```python
from build123d import *

# Parameters (mm, degrees)
SKETCH_1_R          = 5
SKETCH_1_W          = 19.999962028
SKETCH_1_H          = 6.000037038
EXTRUDE_1_DEPTH     = 13
SKETCH_2_R          = 2
CUT_EXTRUDE_1_DEPTH = 36.693120105
SKETCH_3_W          = 1
SKETCH_3_H          = 13
CUT_EXTRUDE_2_DEPTH = 13
FILLET_1_R          = 10


with BuildPart() as part:
    # 草图1 → 凸台-拉伸1 (new body)
    # profile 1 of 10: a face of its own
    with BuildSketch(Plane.XY):
        with BuildLine():
            ThreePointArc((18.008966142, -1.894393619), (10.046238322, 2.288323413), (16.668970702, 8.374337866))
            Line((16.668970702, 8.374337866), (0, 12))
            Line((0, 12), (-16.6689706, 8.374337888))
            ThreePointArc((-16.6689706, 8.374337888), (-12.048865281, 7.282483993), (-10, 3))
            ThreePointArc((-10, 3), (-12.632014098, -1.693043455), (-18.008966133, -1.894393624))
            Line((-18.008966133, -1.894393624), (-9.999981014, -5.999962962))
            Line((-9.999981014, -5.999962962), (9.999981014, -5.999962962))
            Line((9.999981014, -5.999962962), (18.008966142, -1.894393619))
        make_face()
        with Locations(Location((0, 2, 0), (0, 0, 180))):
            Circle(SKETCH_1_R, mode=Mode.SUBTRACT)
    # profile 2 of 10: a face of its own
    with BuildSketch(Plane.XY):
        with BuildLine():
            ThreePointArc((-10, 3), (-12.048865281, 7.282483993), (-16.6689706, 8.374337888))
            ThreePointArc((-16.6689706, 8.374337888), (-18.13580723, 7.827268404), (-19.389087297, 6.889087297))
            Line((-19.389087297, 6.889087297), (-18.680885962, 6.180885962))
            ThreePointArc((-18.680885962, 6.180885962), (-13.778516922, 7.156027793), (-11.001547932, 3))
            ThreePointArc((-11.001547932, 3), (-13.778516922, -1.156027793), (-18.680885962, -0.180885962))
            Line((-18.680885962, -0.180885962), (-19.389087297, -0.889087297))
            ThreePointArc((-19.389087297, -0.889087297), (-18.738276104, -1.445623452), (-18.008966133, -1.894393624))
            ThreePointArc((-18.008966133, -1.894393624), (-12.632014098, -1.693043455), (-10, 3))
        make_face()
    # profile 3 of 10: a face of its own
    with BuildSketch(Plane.XY):
        with BuildLine():
            Line((-18.680885962, 6.180885962), (-19.389087297, 6.889087297))
            ThreePointArc((-19.389087297, 6.889087297), (-20.581337429, 5.104758878), (-21, 3))
            ThreePointArc((-21, 3), (-20.581337429, 0.895241122), (-19.389087297, -0.889087297))
            Line((-19.389087297, -0.889087297), (-18.680885962, -0.180885962))
            ThreePointArc((-18.680885962, -0.180885962), (-19.998452068, 3), (-18.680885962, 6.180885962))
        make_face()
    # profile 4 of 10: a face of its own
    with BuildSketch(Plane.XY):
        with BuildLine():
            ThreePointArc((-10, 3), (-12.048865281, 7.282483993), (-16.6689706, 8.374337888))
            ThreePointArc((-16.6689706, 8.374337888), (-18.13580723, 7.827268404), (-19.389087297, 6.889087297))
            Line((-19.389087297, 6.889087297), (-18.680885962, 6.180885962))
            ThreePointArc((-18.680885962, 6.180885962), (-13.778516922, 7.156027793), (-11.001547932, 3))
            ThreePointArc((-11.001547932, 3), (-13.778516922, -1.156027793), (-18.680885962, -0.180885962))
            Line((-18.680885962, -0.180885962), (-19.389087297, -0.889087297))
            ThreePointArc((-19.389087297, -0.889087297), (-18.738276104, -1.445623452), (-18.008966133, -1.894393624))
            ThreePointArc((-18.008966133, -1.894393624), (-12.632014098, -1.693043455), (-10, 3))
        make_face()
    # profile 5 of 10: a face of its own
    with BuildSketch(Plane.XY):
        with BuildLine():
            Line((-18.680885962, 6.180885962), (-19.389087297, 6.889087297))
            ThreePointArc((-19.389087297, 6.889087297), (-20.581337429, 5.104758878), (-21, 3))
            ThreePointArc((-21, 3), (-20.581337429, 0.895241122), (-19.389087297, -0.889087297))
            Line((-19.389087297, -0.889087297), (-18.680885962, -0.180885962))
            ThreePointArc((-18.680885962, -0.180885962), (-19.998452068, 3), (-18.680885962, 6.180885962))
        make_face()
    # profile 6 of 10: a face of its own
    with BuildSketch(Plane.XY):
        with BuildLine():
            ThreePointArc((18.680885962, -0.180885962), (11.001547932, 3), (18.680885962, 6.180885962))
            Line((18.680885962, 6.180885962), (19.389087297, 6.889087297))
            ThreePointArc((19.389087297, 6.889087297), (18.135807275, 7.82726838), (16.668970702, 8.374337866))
            ThreePointArc((16.668970702, 8.374337866), (10.046238322, 2.288323413), (18.008966142, -1.894393619))
            ThreePointArc((18.008966142, -1.894393619), (18.738276108, -1.445623449), (19.389087297, -0.889087297))
            Line((19.389087297, -0.889087297), (18.680885962, -0.180885962))
        make_face()
    # profile 7 of 10: a face of its own
    with BuildSketch(Plane.XY):
        with BuildLine():
            Line((19.389087297, 6.889087297), (18.680885962, 6.180885962))
            ThreePointArc((18.680885962, 6.180885962), (19.656027793, 4.721483078), (19.998452068, 3))
            ThreePointArc((19.998452068, 3), (19.656027793, 1.278516922), (18.680885962, -0.180885962))
            Line((18.680885962, -0.180885962), (19.389087297, -0.889087297))
            ThreePointArc((19.389087297, -0.889087297), (20.581337429, 0.895241122), (21, 3))
            ThreePointArc((21, 3), (20.581337429, 5.104758878), (19.389087297, 6.889087297))
        make_face()
    # profile 8 of 10: a face of its own
    with BuildSketch(Plane.XY):
        with BuildLine():
            ThreePointArc((18.680885962, -0.180885962), (11.001547932, 3), (18.680885962, 6.180885962))
            Line((18.680885962, 6.180885962), (19.389087297, 6.889087297))
            ThreePointArc((19.389087297, 6.889087297), (18.135807275, 7.82726838), (16.668970702, 8.374337866))
            ThreePointArc((16.668970702, 8.374337866), (10.046238322, 2.288323413), (18.008966142, -1.894393619))
            ThreePointArc((18.008966142, -1.894393619), (18.738276108, -1.445623449), (19.389087297, -0.889087297))
            Line((19.389087297, -0.889087297), (18.680885962, -0.180885962))
        make_face()
    # profile 9 of 10: a face of its own
    with BuildSketch(Plane.XY):
        with BuildLine():
            Line((19.389087297, 6.889087297), (18.680885962, 6.180885962))
            ThreePointArc((18.680885962, 6.180885962), (19.656027793, 4.721483078), (19.998452068, 3))
            ThreePointArc((19.998452068, 3), (19.656027793, 1.278516922), (18.680885962, -0.180885962))
            Line((18.680885962, -0.180885962), (19.389087297, -0.889087297))
            ThreePointArc((19.389087297, -0.889087297), (20.581337429, 0.895241122), (21, 3))
            ThreePointArc((21, 3), (20.581337429, 5.104758878), (19.389087297, 6.889087297))
        make_face()
    # profile 10 of 10: a face of its own
    with BuildSketch(Plane.XY):
        with Locations((0, -8.999981481)):
            Rectangle(SKETCH_1_W, SKETCH_1_H)
    extrude(amount=EXTRUDE_1_DEPTH)

    # 草图2 → 切除-拉伸1 (cut, through all)
    with BuildSketch(Plane.ZY.offset(9.999981014)):
        with Locations((6.487900744, -8.999981481)):
            Circle(SKETCH_2_R)
    extrude(amount=-CUT_EXTRUDE_1_DEPTH, mode=Mode.SUBTRACT)

    # 草图3 → 切除-拉伸2 (cut)
    with BuildSketch(Plane.XZ.offset(12)):
        with Locations((0, 6.5)):
            Rectangle(SKETCH_3_W, SKETCH_3_H)
    extrude(amount=-CUT_EXTRUDE_2_DEPTH, mode=Mode.SUBTRACT)

    # 圆角1
    fillet_1_edges = [part.edges().sort_by_distance(p)[0] for p in [
        (0, 12, 6.5),
    ]]
    fillet(fillet_1_edges, radius=FILLET_1_R)


solid = part.part
```
Verification items for the finished model (mm, model axes). A direction names the side the tool comes from. Round coordinates to 2 decimals unless told otherwise and drop trailing zeros. Order: outer loops, then holes, each group sorted by start corner. A loop starts at its lowest first (then second) coordinate and runs counter-clockwise, first axis right, second up. Notation, with made-up numbers: (-20, 53) - (-16, 53) arc R5 ccw to (-16, 60) - close; hole circle Ø11 at (21, -36). An arc over 180 degrees is marked (long way). Use CSV: the item, a comma, the result in double quotes.
(1) Mould release check, pull along X, two halves, no side actions. Record for faces 1 (the face through (-5, 0, 13)), 2 (the face through (0, 7, 6)), 3 (the face through (13.9, -4, 6.4)): released by +X, released by -X, zero draft, split by the parting line, or undercut.
Entries:
face 1,"zero draft"
face 2,"undercut"
face 3,"released by +X"
(2) Section check D-D on z = 7.75. Record the boundary of the cut face in (x, y).
Entries:
outline,"(-18.01, -1.89) - (-10, -6) - (-10, -7.45) - (-0.5, -7.45) - (-0.5, -2.97) arc R5 cw (long way) to (0.5, -2.97) - (0.5, -7.45) - (10, -7.45) - (10, -6) - (18.01, -1.89) arc R5.5 ccw to (16.67, 8.37) - (2.13, 11.54) arc R10 ccw to (-2.13, 11.54) - (-16.67, 8.37) arc R5.5 ccw to start; (-10, -12) - (-0.5, -12) - (-0.5, -10.55) - (-10, -10.55) - close; (0.5, -12) - (10, -12) - (10, -10.55) - (0.5, -10.55) - close; hole circle Ø9 at (-15.5, 3); hole circle Ø9 at (15.5, 3)"
(3) Section check C-C on x = -11.5. Record the boundary of the cut face in (y, z).
Entries:
outline,"(-5.23, 0) - (0.94, 0) - (0.94, 13) - (-5.23, 13) - close; (5.06, 0) - (9.5, 0) - (9.5, 13) - (5.06, 13) - close"
(4) Section check A-A on z = 2.25. Record the boundary of the cut face in (x, y).
Entries:
outline,"(-18.01, -1.89) - (-10, -6) - (-10, -12) - (-0.5, -12) - (-0.5, -2.97) arc R5 cw (long way) to (0.5, -2.97) - (0.5, -12) - (10, -12) - (10, -6) - (18.01, -1.89) arc R5.5 ccw to (16.67, 8.37) - (2.13, 11.54) arc R10 ccw to (-2.13, 11.54) - (-16.67, 8.37) arc R5.5 ccw to start; hole circle Ø9 at (-15.5, 3); hole circle Ø9 at (15.5, 3)"
(5) Gauge pin test, flat ends, axial feed: pin 1 Ø7 at (y, z) = (-6.5, 7) entering from +X; pin 2 Ø2 at (x, z) = (16.5, 10.5) entering from -Y; pin 3 Ø2 at (x, z) = (11.5, 2.5) entering from -Y; pin 4 Ø4 at (x, y) = (12.5, -5) entering from +Z. Record the tip position at first contact, or that the pin passes through.
Entries:
pin 1,"x = 15.85"
pin 2,"y = -3.18"
pin 3,"y = -5.74"
pin 4,"z = 13"
(6) Section check B-B on y = 2. Record the boundary of the cut face in (x, z).
Entries:
outline,"(-20.91, 0) - (-19.89, 0) - (-19.89, 13) - (-20.91, 13) - close; (-11.11, 0) - (-5, 0) - (-5, 13) - (-11.11, 13) - close; (5, 0) - (11.11, 0) - (11.11, 13) - (5, 13) - close; (19.89, 0) - (20.91, 0) - (20.91, 13) - (19.89, 13) - close"
(7) Thickness scan on probe 1 along Y at (x, z) = (1.5, 6.25); probe 2 along X at (y, z) = (3, 4.5); probe 3 along X at (y, z) = (6.5, 10.5). Record the ranges inside material, lowest first. Write a range as from..to.
Entries:
probe 1,"-12..-10.99, -7.01..-2.77, 6.77..11.65"
probe 2,"-21..-20, -11..-4.9, 4.9..11, 20..21"
probe 3,"-19.74..-18.33, -12.67..-2.18, 2.18..12.67, 18.33..19.74"
(8) Access from +Z, -Z, +X, -X, +Y, -Y to the whole of each face (thin tool, end or side, straight path). Record for faces 4 (the face through (-10, -11, 5)), 5 (the face through (10, -11, 5)), 6 (the face through (-0.5, -6.5, 6.4)), 7 (the face through (5.183, -7.017, 6.228)).
Entries:
face 4,"+Z, -Z, -X, -Y"
face 5,"+Z, -Z, +X, -Y"
face 6,"+Z, -Z, -Y"
face 7,"+X, -X"
